```python
from build123d import *

# Parameters (mm, degrees)
BOSS_EXTRUDE1_DEPTH            = 24
CUT_EXTRUDE1_DEPTH             = 25
SKETCH3_W                      = 7.55
SKETCH3_H                      = 24
F_4_5_4_5_DIAMETER_HOLE1_D     = 4.5
F_4_5_4_5_DIAMETER_HOLE1_DEPTH = 6
CHAMFER1_SIZE                  = 8


with BuildPart() as part:
    # Sketch1 → Boss-Extrude1 (new body)
    with BuildSketch(Plane(origin=(0, 24, 0), x_dir=(1, 0, 0), z_dir=(0, 1, 0))):
        with BuildLine():
            Line((0, 0), (47, 0))
            Line((47, 0), (47, 6))
            Line((47, 6), (38.5, 6))
            ThreePointArc((38.5, 6), (35.307693119, 7.131854655), (33.541354656, 10.021831577))
            ThreePointArc((33.541354656, 10.021831577), (23.505747016, 20.045434485), (13.49594739, 9.996059012))
            ThreePointArc((13.49594739, 9.996059012), (11.698748894, 7.121907302), (8.5, 6))
            Line((8.5, 6), (0, 6))
            Line((0, 6), (0, 0))
        make_face()
    extrude(amount=-BOSS_EXTRUDE1_DEPTH)

    # Sketch2 → Cut-Extrude1 (cut, through all)
    with BuildSketch(Plane.XZ):
        with BuildLine():
            Line((24.018633311, 0), (23.018633311, 0))
            Line((23.018633311, 0), (23.018633311, -2.489295869))
            ThreePointArc((23.018633311, -2.489295869), (23.518633311, -2.472721384), (24.018633311, -2.489295869))
            Line((24.018633311, -2.489295869), (24.018633311, 0))
        make_face()
    extrude(amount=-CUT_EXTRUDE1_DEPTH, mode=Mode.SUBTRACT)

    # Sketch3 → Cut-Revolve1 (revolve, cut)
    with BuildSketch(Plane(origin=(0, 0, -10.022721384), x_dir=(-1, 0, 0), z_dir=(0, 0, -1))):
        with Locations((-27.293633311, 12)):
            Rectangle(SKETCH3_W, SKETCH3_H)
    revolve(axis=Axis((23.518633311, 0, -10.022721384), (0, 1, 0)), mode=Mode.SUBTRACT)

    # Ø4.5 (4.5) Diameter Hole1
    with Locations(Plane(origin=(0, 0, -6), x_dir=(-1, 0, 0), z_dir=(0, 0, -1))):
        with Locations((-41.037266621, 12), (-6, 12)):
            Hole(F_4_5_4_5_DIAMETER_HOLE1_D / 2, depth=F_4_5_4_5_DIAMETER_HOLE1_DEPTH)

    # Chamfer1
    chamfer1_edges = [part.edges().sort_by_distance(p)[0] for p in [
        (47, 0, -3),
        (0, 24, -3),
        (0, 0, -3),
        (47, 24, -3),
    ]]
    chamfer(chamfer1_edges, length=CHAMFER1_SIZE)


solid = part.part
```
CAD build for the part. Positions are in the model's coordinates, mm. A direction names the side the tool comes from. Give positions to 0.01 mm unless a question says otherwise; leave off trailing zeros. Write each loop counter-clockwise with the first axis right and the second up, starting at its lowest first coordinate (ties: lowest second). Pieces come first, ordered by that corner, then holes. Notation, with made-up numbers: M 4.5,79 L 44.5,79 A9 ccw 44.5,92 Z; hole C -36.5,49 d8. An arc over 180 degrees is marked long. Return JSON: item names as keys, results as strings. Group by question number.
(1) Mould opens along Y. For faces 6 (the face through (4, 4, -3)), 7 (the face through (43.18, 12.68, -2.96)), 8 (the face through (11.736, 12.168, -7.152)) say: pulls with the +Y half, pulls with the -Y half, needs draft (parallel to the pull), parting line crosses it, or undercut.
(2) Band-saw the part on C-C (x = 6). Give the cut face in (y, z), and give its area (3 significant figures).
(3) 3-axis set-ups, long thin cutter, end or side, ignore diameter. For faces 1 (the face through (0, 12, -3)), 2 (the face through (24.019, 12, -1)), 3 (the face through (44, 12, -6)), 4 (the face through (3, 12, -6)), 5 (the face through (7.21, 13.897, -2.958)): which of +Z, -Z, +X, -X, +Y, -Y reach the whole face in a straight line?
(4) Band-saw the part on A-A (z = -1.75). Give the cut face in (x, y).
(5) Flat gauge pins, fed straight in: pin 1 Ø5 at (x, y) = (27, 6) entering from -Z; pin 2 Ø12 at (x, y) = (36, 16.5) entering from -Z; pin 3 Ø7 at (x, y) = (6, 12) entering from -Z. Where does each tip first touch, or does it go through?
(6) Drill centre lines: L1, parallel to X at y = 12.5, z = -2; L2, parallel to X at y = 22.25, z = -10.25; L3, parallel to X at y = 14.75, z = -12.75. Where is each one in solid material? Low to high. Write a range as [from, to].
(7) Band-saw the part on B-B (y = 12). Give the cut face in (x, z).
(8) Band-saw the part on D-D (y = 21.5). Give the cut face in (x, z).
Entries:
{
 "1": {"face 6": "pulls with the -Y half", "face 7": "undercut", "face 8": "needs draft"},
 "2": {"outline": "M 2,-6 L 9.75,-6 L 9.75,0 L 2,0 Z; M 14.25,-6 L 22,-6 L 22,0 L 14.25,0 Z", "area": "93.0 mm^2"},
 "3": {"face 1": "+Z, -Z, -X, +Y, -Y", "face 2": "+Z, +Y, -Y", "face 3": "-Z, +X, +Y, -Y", "face 4": "-Z, -X, +Y, -Y", "face 5": "+Z, -Z"},
 "4": {"outline": "M 0,8 L 8,0 L 23.02,0 L 23.02,24 L 8,24 L 0,16 Z; M 24.02,0 L 39,0 L 47,8 L 47,16 L 39,24 L 24.02,24 Z; hole C 6,12 d4.5; hole C 41.04,12 d4.5"},
 "5": {"pin 1": "stops at z = -20", "pin 2": "stops at z = -17.67", "pin 3": "stops at z = -6.1"},
 "6": {"L1": "x = [0, 3.81], [8.19, 23.02], [24.02, 38.84], [43.23, 47]", "L2": "x = [13.5, 15.97], [31.07, 33.54]", "L3": "x = [13.87, 16.48], [30.56, 33.16]"},
 "7": {"outline": "M 0,-6 L 3.75,-6 L 3.75,0 L 0,0 Z; M 8.25,-6 L 8.5,-6 A5.12 cw 13.5,-10 A10.02 ccw 33.54,-10.02 A5.07 cw 38.5,-6 L 38.79,-6 L 38.79,0 L 24.02,0 L 24.02,-2.49 A7.55 cw long 23.02,-2.49 L 23.02,0 L 8.25,0 Z; M 43.29,-6 L 47,-6 L 47,0 L 43.29,0 Z"},
 "8": {"outline": "M 5.5,-6 L 8.5,-6 A5.12 cw 13.5,-10 A10.02 ccw 33.54,-10.02 A5.07 cw 38.5,-6 L 41.5,-6 L 41.5,0 L 24.02,0 L 24.02,-2.49 A7.55 cw long 23.02,-2.49 L 23.02,0 L 5.5,0 Z"}
}
